Input: part model. Units: mm. Frame: model coordinates. A direction names the side the tool comes from. Give positions to 0.01 mm unless a question says otherwise; leave off trailing zeros. Write each loop counter-clockwise with the first axis right and the second up, starting at its lowest first coordinate (ties: lowest second). Pieces come first, ordered by that corner, then holes. Notation, with made-up numbers: (49, 74.5) - (106, 74.5) arc R18 ccw to (106, 88.5) - close; hole circle Ø6 at (65.25, 45). An arc over 180 degrees is marked (long way). Answer as CSV lines item,"result".
```python
from build123d import *

# Parameters (mm, degrees)
F0_W     = 300
F0_H     = 175
F1_DEPTH = 30
F2_W     = 9.5
F2_H     = 165
F3_DEPTH = 39.5


with BuildPart() as f1:
    # F0 (on Front) → F1 (new body)
    with BuildSketch(Plane.XZ):
        Rectangle(F0_W, F0_H)
    extrude(amount=F1_DEPTH)

    # F2 (on face) → F3 (join)
    with BuildSketch(Plane.YZ.offset(150)):
        with Locations((-15, 0.5)):
            Rectangle(F2_W, F2_H)
    extrude(amount=F3_DEPTH)


solid = f1.part
```
Item 1: Reachability of faces 1 (the face through (169, -15, -82)), 2 (the face through (169, -19.75, -1)), 3 (the face through (169, -15, 83)), 4 (the face through (169, -10.25, -1)) from +Z, -Z, +X, -X, +Y, -Y: full face, straight path, thin tool, end or side. Return the list, or none.
The answers:
face 1,"-Z, +X, +Y, -Y"
face 2,"+Z, -Z, +X, -Y"
face 3,"+Z, +X, +Y, -Y"
face 4,"+Z, -Z, +X, +Y"
Item 2: Cut plane B-B on y = -26.5. Return the cut outline in (x, z).
The answers:
outline,"(-150, -87.5) - (150, -87.5) - (150, 87.5) - (-150, 87.5) - close"
Item 3: Cut plane A-A on z = -25. Return the cut outline in (x, y), plus the area to 3 significant figures.
The answers:
outline,"(-150, -30) - (150, -30) - (150, -19.75) - (189.5, -19.75) - (189.5, -10.25) - (150, -10.25) - (150, 0) - (-150, 0) - close"
area,"9,380 mm²"
Item 4: Ray query, line 1 (X direction, y = -28.5, z = 6); line 2 (Z direction, x = 152, y = -15.25). Return the intervals inside material, ascending. Write a range as from..to.
The answers:
line 1,"-150..150"
line 2,"-82..83"
Item 5: Contact query for flat-ended pins moving along their axis: pin 1 (6 mm diameter, centred on x = -36, z = -69, fed in from +Y); pin 2 (5 mm diameter, centred on x = 164, y = -14.5, fed in from +Z); pin 3 (7.5 mm diameter, centred on x = 165.5, y = -15.5, fed in from -Z). Output: stop coordinate, or through.
The answers:
pin 1,"y = 0"
pin 2,"z = 83"
pin 3,"z = -82"
